from build123d import *

# Parameters (mm, degrees)
F0_W     = 120
F0_H     = 120
F0_R     = 2.75
F1_DEPTH = 10


with BuildPart() as f1:
    # F0 (on Top) → F1 (new body)
    with BuildSketch(Plane.XY):
        Rectangle(F0_W, F0_H)
        with Locations((-46, -46)):
            Circle(F0_R, mode=Mode.SUBTRACT)
        with Locations((46, -46)):
            Circle(F0_R, mode=Mode.SUBTRACT)
        with Locations((-46, 46)):
            Circle(F0_R, mode=Mode.SUBTRACT)
        with BuildLine():
            ThreePointArc((4.681734, 44.755797), (33.4341, 30.119113), (45, 0))
            ThreePointArc((45, 0), (-30.119113, -33.4341), (-4.681734, 44.755797))
            ThreePointArc((-4.681734, 44.755797), (0, 45), (4.681734, 44.755797))
        make_face(mode=Mode.SUBTRACT)
        with Locations((46, 46)):
            Circle(F0_R, mode=Mode.SUBTRACT)
    extrude(amount=F1_DEPTH)


solid = f1.part
The model under review builds one solid part; all positions refer to its coordinate system, in mm. Give positions to 0.01 mm unless a question says otherwise; leave off trailing zeros. Order: outer loops, then holes, each group sorted by start corner. A loop starts at its lowest first (then second) coordinate and runs counter-clockwise, first axis right, second up. Notation, with made-up numbers: (7, 61.5) -> (23, 61.5) arc R17 ccw to (23, 70.5) -> close; hole circle Ø11 at (-18.75, 61). An arc over 180 degrees is marked (long way). Write item = value, one per line. Start each with the question number.
(1) Take a section at A-A (z = 8). Write out the cut boundary in (x, y).
(2) Draft analysis for pull direction Y (two halves, no side actions). For faces 1 (the flat face through (-1, -60, 5)), 2 (the flat face through (-1, 60, 5)), 3 (the flat face through (60, -1, 5)), 4 (the cylindrical face through (43.973, 47.859, 4.93)), state which applies: +Y half, -Y half, draft (parallel to the pull), parting line (faces both ways), or undercut.
(3) For L1, parallel to Y at x = -46, z = 6; L2, parallel to X at y = 47, z = 1.5; L3, parallel to Y at x = -0.5, z = 5.25, list the stretches that pass through material, from the lowest coordinate up. Write a range as from..to.
(4) Take a section at C-C (y = -19). Write out the cut boundary in (x, z), plus the area to 3 significant figures.
(5) For pin 1 Ø1 at (x, y) = (-48, -35.5) entering from -Z, flat-tipped, find the tip position at first contact; note if it passes through.
(6) Take a section at B-B (x = 0). Write out the cut boundary in (y, z).
Returned:
q1.outline = (-60, -60) -> (60, -60) -> (60, 60) -> (-60, 60) -> close; hole circle Ø5.5 at (-46, -46); hole circle Ø5.5 at (-46, 46); hole (-4.68, 44.76) arc R45 ccw (long way) to (4.68, 44.76) arc R45 ccw to start; hole circle Ø5.5 at (46, -46); hole circle Ø5.5 at (46, 46)
q2.face_1 = -Y half
q2.face_2 = +Y half
q2.face_3 = draft
q2.face_4 = undercut
q3.L1 = -60..-48.75, -43.25..43.25, 48.75..60
q3.L2 = -60..-48.56, -43.44..43.44, 48.56..60
q3.L3 = -60..-45, 45..60
q4.outline = (-60, 0) -> (-40.79, 0) -> (-40.79, 10) -> (-60, 10) -> close; (40.79, 0) -> (60, 0) -> (60, 10) -> (40.79, 10) -> close
q4.area = 384 mm²
q5.pin_1 = 0
q6.outline = (-60, 0) -> (-45, 0) -> (-45, 10) -> (-60, 10) -> close; (45, 0) -> (60, 0) -> (60, 10) -> (45, 10) -> close
